from build123d import *

# Parameters (mm, degrees)
SKETCH1_R           = 3
BOSS_EXTRUDE1_DEPTH = 6.35


with BuildPart() as part:
    # Sketch1 → Boss-Extrude1 (new body)
    with BuildSketch(Plane.XY.offset(36.015266699)):
        with BuildLine():
            Line((-1.608835655, 1.421229345), (-31.608835655, 1.421229345))
            ThreePointArc((-31.608835655, 1.421229345), (-44.108835655, 13.921229345), (-31.608835655, 26.421229345))
            Line((-31.608835655, 26.421229345), (-1.608835655, 26.421229345))
            Line((-1.608835655, 26.421229345), (-1.608835655, 1.421229345))
        make_face()
        with Locations((-31.608835655, 13.921229345)):
            Circle(SKETCH1_R, mode=Mode.SUBTRACT)
    extrude(amount=BOSS_EXTRUDE1_DEPTH)


solid = part.part
Model file for the job. Use its own axes, mm. Give positions to 0.01 mm unless a question says otherwise; leave off trailing zeros. Order: outer loops, then holes, each group sorted by start corner. A loop starts at its lowest first (then second) coordinate and runs counter-clockwise, first axis right, second up. Notation, with made-up numbers: (14.25, 47.5) - (59.25, 47.5) arc R20 ccw to (59.25, 79.5) - close; hole circle Ø7 at (27.25, -17). An arc over 180 degrees is marked (long way). Write item = value, one per line. Start each with the question number.
1. Cut at D-D, the plane y = 18.25. List the corners of the cut face in (x, z).
2. Drop a flat-ended pin along its axis: P1, Ø5, axis at x = -31.61, y = 13.92, coming from the -Z side. Give the stop position or say it passes through.
3. Probe line 1 along Y through (x, z) = (-33.5, 38.5); line 2 along X through (y, z) = (14, 36.5); line 3 along X through (y, z) = (19.75, 42). List the from-to ranges inside material, lowest first.
4. Two-plate mould, pull along X, no slides. Class faces 1 (the flat face through (-1.609, 14, 39)), 2 (the flat face through (-23, 14, 36.015)), 3 (the cylindrical face through (-44.106, 13.646, 39.146)), 4 (the cylindrical face through (-28.747, 14.822, 39.146)): pulls with the +X half, pulls with the -X half, needs draft (parallel to the pull), parting line crosses it, or undercut.
5. Cut at A-A, the plane y = 12.5. List the corners of the cut face in (x, z), and give its area (3 significant figures).
6. Cut at C-C, the plane x = -36.5. List the corners of the cut face in (y, z).
7. Cut at B-B, the plane z = 36.5. List the corners of the cut face in (x, y), and give its area (3 significant figures).
Taken from the geometry:
q1.outline = (-43.34, 36.02) - (-1.61, 36.02) - (-1.61, 42.37) - (-43.34, 42.37) - close
q2.P1 = through
q3.line_1 = 1.57 to 11.59, 16.25 to 26.28
q3.line_2 = -44.11 to -34.61, -28.61 to -1.61
q3.line_3 = -42.67 to -1.61
q4.face_1 = pulls with the +X half
q4.face_2 = needs draft
q4.face_3 = pulls with the -X half
q4.face_4 = undercut
q5.outline = (-44.03, 36.02) - (-34.25, 36.02) - (-34.25, 42.37) - (-44.03, 42.37) - close; (-28.97, 36.02) - (-1.61, 36.02) - (-1.61, 42.37) - (-28.97, 42.37) - close
q5.area = 236 mm²
q6.outline = (2.42, 36.02) - (25.42, 36.02) - (25.42, 42.37) - (2.42, 42.37) - close
q7.outline = (-31.61, 1.42) - (-1.61, 1.42) - (-1.61, 26.42) - (-31.61, 26.42) arc R12.5 ccw to start; hole circle Ø6 at (-31.61, 13.92)
q7.area = 967 mm²
